Source: CAD feature listing. Evaluate the final solid. Frame: model axes, mm. Give positions to 0.01 mm unless a question says otherwise; leave off trailing zeros. Order: outer loops, then holes, each group sorted by start corner. A loop starts at its lowest first (then second) coordinate and runs counter-clockwise, first axis right, second up. Notation, with made-up numbers: M 48.5,61 L 90.5,61 A17 ccw 90.5,84 Z; hole C -24,-3 d5. An arc over 180 degrees is marked long. Answer as a JSON object with one key per item and string values. Group by question number.
1. Pin query (flat end, axial travel): P1, Ø4, axis at x = -13.72, y = -76.75, coming from the -Z side; P2, Ø5.5, axis at x = -13.716, y = 88.9, coming from the -Z side. Return the tip coordinate at first contact, or that it passes through.
2. Section query A-A (y = 88.9). Output: boundary loops of the cut face in (x, z) (3 decimals), plus the area to 3 significant figures.
3. Section query B-B (z = 0.6). Output: boundary loops of the cut face in (x, y), plus the area to 3 significant figures.
4. Material intervals for L1, parallel to Y at x = -15.75, z = 2.3; L2, parallel to Y at x = -12.25, z = 2.9; L3, parallel to X at y = 90, z = 0.35, sorted ascending. Write a range as [from, to].
5. Pull-direction query (Y, two-part tool) for faces 1 (the flat face through (-14, -101.6, 2)), 2 (the flat face through (-8.382, -1, 2)), 3 (the cylindrical face through (-16.015, 87.947, 1.565)); classes: +Y half, -Y half, draft (parallel to the pull), parting line (faces both ways), or undercut.
from build123d import *

# Parameters (mm, degrees)
SKETCH1_W              = 10.668
SKETCH1_H              = 203.2
BOSS_EXTRUDE1_DEPTH    = 3.175
F_10_CLEARANCE_HOLE1_D = 4.9784
F_10_CLEARANCE_HOLE2_D = 4.9784


with BuildPart() as part:
    # Sketch1 → Boss-Extrude1 (new body)
    with BuildSketch(Plane.XY):
        with Locations((-13.716, 0)):
            Rectangle(SKETCH1_W, SKETCH1_H)
    extrude(amount=BOSS_EXTRUDE1_DEPTH)

    # #10 Clearance Hole1 (through all)
    with Locations(Plane.XY.offset(3.175)):
        with Locations((-13.716, -76.754256991)):
            Hole(F_10_CLEARANCE_HOLE1_D / 2)

    # #10 Clearance Hole2 (through all)
    with Locations(Plane.XY.offset(3.175)):
        with Locations((-13.716, 88.9)):
            Hole(F_10_CLEARANCE_HOLE2_D / 2)


solid = part.part
Answer sheet:
{
 "1": {"P1": "through", "P2": "z = 0"},
 "2": {"outline": "M -19.05,0 L -16.205,0 L -16.205,3.175 L -19.05,3.175 Z; M -11.227,0 L -8.382,0 L -8.382,3.175 L -11.227,3.175 Z", "area": "18.1 mm^2"},
 "3": {"outline": "M -19.05,-101.6 L -8.38,-101.6 L -8.38,101.6 L -19.05,101.6 Z; hole C -13.72,-76.75 d4.98; hole C -13.72,88.9 d4.98", "area": "2,130 mm^2"},
 "4": {"L1": "[-101.6, -78.19], [-75.32, 87.47], [90.33, 101.6]", "L2": "[-101.6, -78.77], [-74.74, 86.89], [90.91, 101.6]", "L3": "[-19.05, -15.95], [-11.48, -8.38]"},
 "5": {"face 1": "-Y half", "face 2": "draft", "face 3": "undercut"}
}
